Verification items for the finished model (mm, model axes). A direction names the side the tool comes from. Coordinates: 2 decimals unless noted, no trailing zeros. Order: outer loops, then holes, each group sorted by start corner. A loop starts at its lowest first (then second) coordinate and runs counter-clockwise, first axis right, second up. Notation, with made-up numbers: M 22,2.25 L 77,2.25 A21 ccw 77,8.25 Z; hole C 68,31.25 d8. An arc over 180 degrees is marked long. Return JSON: item names as keys, results as strings. Group by question number.
Q1. Section check C-C, the plane x = 23. Enter the section's corners in (y, z).
Q2. Section check A-A, the plane z = 20. Enter the section's corners in (x, y).
Q3. Thickness scan on probe 1 along X at (y, z) = (6, -124); probe 2 along X at (y, z) = (39, -9.5); probe 3 along Z at (x, y) = (116, 37). Record the ranges inside material, lowest first.
Q4. Section check B-B, the plane y = 68. Enter the section's corners in (x, z).
Q5. Access from +Z, -Z, +X, -X, +Y, -Y to the whole of each face (thin tool, end or side, straight path). Record for faces 4 (the face through (-10, 65, -51)), 5 (the face through (23, 85, -109)), 6 (the face through (74, 65, -114)), 7 (the face through (74, 75, -104)).
Q6. Go/stop test with flat-tipped pins: pin 1 Ø1 at (x, y) = (152.5, 86) entering from +Z; pin 2 Ø8 at (y, z) = (109.5, -110.5) entering from -X; pin 3 Ø11.5 at (x, z) = (167.2, 20) entering from +Y. Record where each tip stops, or that it passes through.
Q7. Section check D-D, the plane z = -109. Enter the section's corners in (x, y), then the cut area to 3 significant figures.
Q8. Mould release check, pull along Z, two halves, no side actions. Record for faces 1 (the face through (74, 75, 0)), 2 (the face through (74, 65, 10)), 3 (the face through (37, 111, -109)): pulls with the +Z half, pulls with the -Z half, needs draft (parallel to the pull), parting line crosses it, or undercut.
from build123d import *

# Parameters (mm, degrees)
SKETCH1_W           = 150
SKETCH1_H           = 104
BOSS_EXTRUDE1_DEPTH = 30
SKETCH2_W           = 170
SKETCH2_H           = 124
SKETCH2_W_2         = 150
SKETCH2_H_2         = 104
BOSS_EXTRUDE2_DEPTH = 122
CUT_EXTRUDE2_DEPTH  = 10
SKETCH6_W           = 210
SKETCH6_H           = 164
SKETCH6_R           = 5
BOSS_EXTRUDE3_DEPTH = 10


with BuildPart() as part:
    # Sketch1 → Boss-Extrude1 (new body)
    with BuildSketch(Plane(origin=(0, 0, 0), x_dir=(1, 0, 0), z_dir=(0, 1, 0))):
        with Locations((75, 52)):
            Rectangle(SKETCH1_W, SKETCH1_H)
    extrude(amount=BOSS_EXTRUDE1_DEPTH)

    # Sketch2 → Boss-Extrude2 (add)
    with BuildSketch(Plane(origin=(0, 0, 0), x_dir=(1, 0, 0), z_dir=(0, 1, 0))):
        with Locations((75, 52)):
            Rectangle(SKETCH2_W, SKETCH2_H)
        with Locations((75, 52)):
            Rectangle(SKETCH2_W_2, SKETCH2_H_2, mode=Mode.SUBTRACT)
    extrude(amount=BOSS_EXTRUDE2_DEPTH)

    # Sketch5 → Cut-Extrude2 (cut)
    with BuildSketch(Plane(origin=(0, 0, -114), x_dir=(-1, 0, 0), z_dir=(0, 0, -1))):
        with BuildLine():
            Line((-37, 122), (-37, 99))
            ThreePointArc((-37, 99), (-23, 85), (-9, 99))
            Line((-9, 99), (-9, 122))
            Line((-9, 122), (-37, 122))
        make_face()
    extrude(amount=-CUT_EXTRUDE2_DEPTH, mode=Mode.SUBTRACT)

    # Sketch6 → Boss-Extrude3 (add)
    with BuildSketch(Plane(origin=(0, 0, 0), x_dir=(1, 0, 0), z_dir=(0, 1, 0))):
        with Locations((75, 52)):
            Rectangle(SKETCH6_W, SKETCH6_H)
        with Locations(Location((-17.195121951, -20, 0), (0, 0, 270))):
            Circle(SKETCH6_R, mode=Mode.SUBTRACT)
        with Locations(Location((167.195121951, -20, 0), (0, 0, 270))):
            Circle(SKETCH6_R, mode=Mode.SUBTRACT)
        with Locations(Location((167.195121951, 124, 0), (0, 0, 270))):
            Circle(SKETCH6_R, mode=Mode.SUBTRACT)
        with Locations(Location((-17.195121951, 124, 0), (0, 0, 270))):
            Circle(SKETCH6_R, mode=Mode.SUBTRACT)
    extrude(amount=BOSS_EXTRUDE3_DEPTH)


solid = part.part
Numbers:
{
 "1": {"outline": "M 0,-134 L 10,-134 L 10,-114 L 85,-114 L 85,-104 L 30,-104 L 30,0 L 122,0 L 122,10 L 10,10 L 10,30 L 0,30 Z"},
 "2": {"outline": "M -30,0 L -22.2,0 L -22.2,10 L -30,10 Z; M -12.2,0 L 162.2,0 L 162.2,10 L -12.2,10 Z; M 172.2,0 L 180,0 L 180,10 L 172.2,10 Z"},
 "3": {"probe 1": "x = -30 to -22.2, -12.2 to 162.2, 172.2 to 180", "probe 2": "x = -10 to 0, 150 to 160", "probe 3": "z = -114 to -104, 0 to 10"},
 "4": {"outline": "M -10,-114 L 160,-114 L 160,10 L -10,10 Z; hole M 0,-104 L 150,-104 L 150,0 L 0,0 Z"},
 "5": {"face 4": "+Z, -Z, -X, +Y", "face 5": "-Z, +Y", "face 6": "-Z, +X, -X, +Y", "face 7": "+Y"},
 "6": {"pin 1": "stops at z = 10", "pin 2": "stops at x = -10", "pin 3": "stops at y = 10"},
 "7": {"outline": "M -30,0 L 180,0 L 180,10 L 160,10 L 160,122 L 37,122 L 37,99 A14 cw 9,99 L 9,122 L -10,122 L -10,10 L -30,10 Z", "area": "20,200 mm2"},
 "8": {"face 1": "undercut", "face 2": "pulls with the +Z half", "face 3": "needs draft"}
}
